Can you work these out from the model? Positions are in its coordinate system, mm. Face numbers are marked on the shaded views. A direction names the side the tool comes from. Coordinates: 2 decimals unless noted, no trailing zeros. Write each loop counter-clockwise with the first axis right and the second up, starting at its lowest first coordinate (ties: lowest second). Pieces come first, ordered by that corner, then holes. Notation, with made-up numbers: (19.5, -24) - (54.5, -24) arc R7 cw to (54.5, -18) - close; hole circle Ø5 at (69.25, -18.75). An arc over 180 degrees is marked (long way). Use one line per item in the form item = value. Start each with the question number.
(1) On a 3-axis mill with a long thin cutter (end or side, diameter ignored), from which of +Z, -Z, +X, -X, +Y, -Y can I reach the whole of each face in a straight line? I mean the marked faces 1, 2 and 3. Say none if no direction works.
(2) If I drill on probe 1 along Y at (x, z) = (0, -1); probe 2 along Z at (x, y) = (0.5, -11.5); probe 3 along Y at (x, z) = (-2, -0.5), over which ranges is the centre line in solid material (lowest first)? Write a range as from..to.
(3) Thinking about a two-plate mould opening in X: for the marked faces 4, 5 and 6, which applies, pulls with the +X half, pulls with the -X half, needs draft (parallel to the pull), parting line crosses it, or undercut?
(4) For pin 1 Ø3 at (y, z) = (1, 6) entering from +X; pin 2 Ø5.5 at (x, y) = (1.5, -1.5) entering from +Z; pin 3 Ø2.5 at (y, z) = (2.5, -4.5) entering from +X, each with a flat end and sliding along its axis, tell me the tip position at first contact or that it passes through.
(5) If we section it at A-A on z = -1: Please give me the cut outline in (x, y), then the cut area to 3 significant figures.
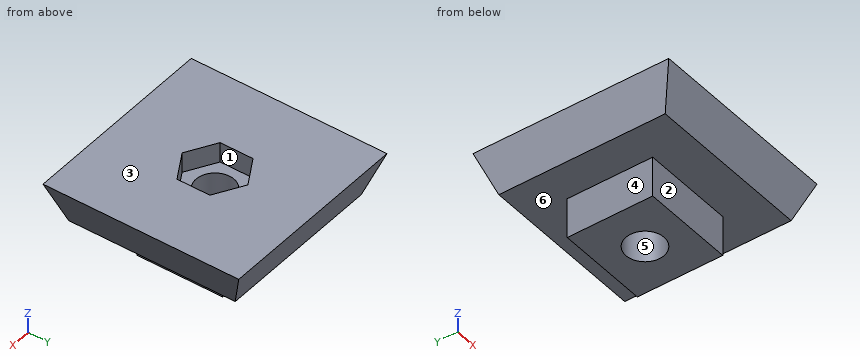
```python
from build123d import *

# Parameters (mm, degrees)
F0_W     = 33
F0_H     = 33
F1_DEPTH = 8
F1_TAPER = -20
F3_DEPTH = 4
F4_W     = 18.3548238128
F4_H     = 16.941415146
F5_DEPTH = 8
F7_D     = 7.5438
F7_DEPTH = 25
F7_TIP   = 2.2663861689


with BuildPart() as f1:
    # F0 (on Top) → F1 (new body)
    with BuildSketch(Plane.XY):
        Rectangle(F0_W, F0_H)
    extrude(amount=F1_DEPTH, taper=F1_TAPER)

    # F2 (on face) → F3 (cut)
    with BuildSketch(Plane.XY.offset(8)):
        Polygon((5.65, -3.2620290209), (5.65, 3.2620290209), (0, 6.5240580418), (-5.65, 3.2620290209), (-5.65, -3.2620290209), (0, -6.5240580418), align=None)
    extrude(amount=-F3_DEPTH, mode=Mode.SUBTRACT)

    # F4 (on face) → F5 (join)
    with BuildSketch(Plane(origin=(0, 0, 0), x_dir=(1, 0, 0), z_dir=(0, 0, -1))):
        Rectangle(F4_W, F4_H)
    extrude(amount=F5_DEPTH)

    # F7
    with Locations(Plane(origin=(0, 0, -8), x_dir=(1, 0, 0), z_dir=(0, 0, -1))):
        with Locations((0, 0)):
            Hole(F7_D / 2, depth=F7_DEPTH)
            with Locations((0, 0, -(F7_DEPTH + F7_TIP / 2))):  # 118° drill point
                Cone(0, F7_D / 2, F7_TIP, mode=Mode.SUBTRACT)


solid = f1.part
```
Reported:
q1.face_1 = +Z
q1.face_2 = -Z, +X, -X, -Y
q1.face_3 = +Z, +X, -X, +Y, -Y
q2.probe_1 = -8.47..-3.77, 3.77..8.47
q2.probe_2 = 0..8
q2.probe_3 = -8.47..-3.2, 3.2..8.47
q3.face_4 = pulls with the -X half
q3.face_5 = undercut
q3.face_6 = needs draft
q4.pin_1 = 19.23
q4.pin_2 = 4
q4.pin_3 = 9.18
q5.outline = (-9.18, -8.47) - (9.18, -8.47) - (9.18, 8.47) - (-9.18, 8.47) - close; hole circle Ø7.54 at (0, 0)
q5.area = 266 mm2
